The listing builds one solid part. Answer for the finished solid, in the listing's coordinates (mm). A direction names the side the tool comes from. Give positions to 0.01 mm unless a question says otherwise; leave off trailing zeros. Write each loop counter-clockwise with the first axis right and the second up, starting at its lowest first coordinate (ties: lowest second). Pieces come first, ordered by that corner, then holes.
```python
from build123d import *

# Parameters (mm, degrees)
F2_W      = 39
F2_H      = 30
F3_DEPTH  = 1
F5_DEPTH  = 4
F8_DEPTH  = 4
F11_DEPTH = 4
F14_DEPTH = 4
F17_DEPTH = 4
F20_DEPTH = 4


with BuildPart() as f3:
    # F2 (on Top) → F3 (new body)
    with BuildSketch(Plane.XY):
        Rectangle(F2_W, F2_H)
    extrude(amount=F3_DEPTH)

    # F4 (on face) → F5 (join)
    with BuildSketch(Plane(origin=(-19.5, 0, 0), x_dir=(0, -1, 0), z_dir=(-1, 0, 0))):
        Polygon((5.5351936674, 1), (15, 1), (-12.1892336111, 13.6785478522), (-13.8797066581, 10.0533167041), align=None)
    extrude(amount=-F5_DEPTH)

    # F7 (on offset) → F8 (join)
    with BuildSketch(Plane.YZ.offset(-12.5)):
        Polygon((-15, 1), (-7, 1), (12.9807621135, 12.5358983849), (10.9807621135, 16), align=None)
    extrude(amount=F8_DEPTH)

    # F10 (on offset) → F11 (join)
    with BuildSketch(Plane.YZ.offset(-5.5)):
        Polygon((9.5745613287, 18.2072930905), (-15, 1), (-8.0262128175, 1), (11.8688670741, 14.9306849134), align=None)
    extrude(amount=F11_DEPTH)

    # F13 (on offset) → F14 (join)
    with BuildSketch(Plane.YZ.offset(1.5)):
        Polygon((7.9813332936, 20.2836282906), (-15, 1), (-8.7771046926, 1), (10.5524837323, 17.2194505181), align=None)
    extrude(amount=F14_DEPTH)

    # F16 (on offset) → F17 (join)
    with BuildSketch(Plane.YZ.offset(8.5)):
        Polygon((6.2132034356, 22.2132034356), (-15, 1), (-9.3431457505, 1), (9.0416305603, 19.3847763109), align=None)
    extrude(amount=F17_DEPTH)

    # F19 (on offset) → F20 (join)
    with BuildSketch(Plane.YZ.offset(15.5)):
        Polygon((4.2836282906, 23.9813332936), (-15, 1), (-9.7783708427, 1), (7.3478060631, 21.4101828548), align=None)
    extrude(amount=F20_DEPTH)


solid = f3.part
```
Item 1: Consider probe 1 along X at (y, z) = (4.25, 16); probe 2 along X at (y, z) = (4, 19.25); probe 3 along X at (y, z) = (-0.5, 10.25). Determine where each line is inside the solid, lowest interval first.
Conclusion:
probe 1: x = 1.5 to 5.5, 8.5 to 12.5
probe 2: x = 8.5 to 12.5, 15.5 to 19.5
probe 3: x = -5.5 to -1.5, 1.5 to 5.5, 8.5 to 12.5
Item 2: Each of these flat-tipped pins is pushed along its axis until it touches: P1, Ø4, axis at y = 6, z = 8.5, coming from the +X side; P2, Ø5, axis at x = -11.5, y = -9.5, coming from the +Z side; P3, Ø6.5, axis at y = -5.5, z = 17, coming from the -X side. Where does it stop, or does it pass through?
Conclusion:
P1: stops at x = -1.5
P2: stops at z = 5.62
P3: stops at x = 15.5
Item 3: A cutting plane is placed at D-D, the plane y = 1.5. Give the vertices of the cut face in (x, z).
Conclusion:
outline: (-19.5, 0) - (19.5, 0) - (19.5, 1) - (-19.5, 1) - close; (-19.5, 4.28) - (-15.5, 4.28) - (-15.5, 8.69) - (-19.5, 8.69) - close; (-12.5, 5.91) - (-8.5, 5.91) - (-8.5, 10.53) - (-12.5, 10.53) - close; (-5.5, 7.67) - (-1.5, 7.67) - (-1.5, 12.55) - (-5.5, 12.55) - close; (1.5, 9.62) - (5.5, 9.62) - (5.5, 14.85) - (1.5, 14.85) - close; (8.5, 11.84) - (12.5, 11.84) - (12.5, 17.5) - (8.5, 17.5) - close; (15.5, 14.44) - (19.5, 14.44) - (19.5, 20.66) - (15.5, 20.66) - close
Item 4: A cutting plane is placed at A-A, the plane z = 6. Give the vertices of the cut face in (x, y), plus the area to 3 significant figures.
Conclusion:
outline: (-19.5, -4.28) - (-15.5, -4.28) - (-15.5, 5.19) - (-19.5, 5.19) - close; (-12.5, -6.34) - (-8.5, -6.34) - (-8.5, 1.66) - (-12.5, 1.66) - close; (-5.5, -7.86) - (-1.5, -7.86) - (-1.5, -0.89) - (-5.5, -0.89) - close; (1.5, -9.04) - (5.5, -9.04) - (5.5, -2.82) - (1.5, -2.82) - close; (8.5, -10) - (12.5, -10) - (12.5, -4.34) - (8.5, -4.34) - close; (15.5, -10.8) - (19.5, -10.8) - (19.5, -5.58) - (15.5, -5.58) - close
area: 166 mm2
Item 5: A cutting plane is placed at B-B, the plane x = -9. Give the vertices of the cut face in (y, z), plus the area to 3 significant figures.
Conclusion:
outline: (-15, 0) - (15, 0) - (15, 1) - (-7, 1) - (12.98, 12.54) - (10.98, 16) - (-15, 1) - close
area: 136 mm2
Item 6: Determine the mould class of faces 5 (the face through (19.5, -3, 11)), 6 (the face through (1.5, -1, 10)), 7 (the face through (17.472, 5.837, 22.678)) for opening direction X: pulls with the +X half, pulls with the -X half, needs draft (parallel to the pull), parting line crosses it, or undercut.
Conclusion:
face 5: pulls with the +X half
face 6: undercut
face 7: needs draft
Item 7: Which of the six approach directions +Z, -Z, +X, -X, +Y, -Y give full straight-line access (tool end or side, diameter ignored) to faces 1 (the face through (3.472, -3.348, 10.777)), 2 (the face through (-1.5, -1, 9)), 3 (the face through (-17.528, 13.023, 11.891)), 4 (the face through (3.472, 0.752, 8.996))?
Conclusion:
face 1: +Z, -X, -Y
face 2: +Z, +Y, -Y
face 3: +Z, -X, +Y
face 4: +X, +Y
Item 8: A cutting plane is placed at C-C, the plane z = 18.75. Give the vertices of the cut face in (x, y), plus the area to 3 significant figures.
Conclusion:
outline: (1.5, 6.15) - (5.5, 6.15) - (5.5, 9.27) - (1.5, 9.27) - close; (8.5, 2.75) - (12.5, 2.75) - (12.5, 8.41) - (8.5, 8.41) - close; (15.5, -0.11) - (19.5, -0.11) - (19.5, 5.12) - (15.5, 5.12) - close
area: 56.0 mm2
